from build123d import *

# Parameters (mm, degrees)
BOSS_EXTRUDE2_DEPTH = 18
SKETCH7_W           = 24
SKETCH7_H           = 13
CUT_EXTRUDE8_DEPTH  = 16.5


with BuildPart() as part:
    # Sketch2 → Boss-Extrude2 (new body)
    with BuildSketch(Plane(origin=(0, 0, 0), x_dir=(1, 0, 0), z_dir=(0, 1, 0))):
        with BuildLine():
            Line((14.142135624, 0), (48.904069139, 34.761933515))
            ThreePointArc((48.904069139, 34.761933515), (42.426406871, 42.426406871), (34.761933515, 48.904069139))
            Line((34.761933515, 48.904069139), (0, 14.142135624))
            Line((0, 14.142135624), (-34.761933515, 48.904069139))
            ThreePointArc((-34.761933515, 48.904069139), (-42.426406871, 42.426406871), (-48.904069139, 34.761933515))
            Line((-48.904069139, 34.761933515), (-14.142135624, 0))
            Line((-14.142135624, 0), (-48.904069139, -34.761933515))
            ThreePointArc((-48.904069139, -34.761933515), (-42.426406871, -42.426406871), (-34.761933515, -48.904069139))
            Line((-34.761933515, -48.904069139), (0, -14.142135624))
            Line((0, -14.142135624), (34.761933515, -48.904069139))
            ThreePointArc((34.761933515, -48.904069139), (42.426406871, -42.426406871), (48.904069139, -34.761933515))
            Line((48.904069139, -34.761933515), (14.142135624, 0))
        make_face()
    extrude(amount=BOSS_EXTRUDE2_DEPTH)

    # Sketch7 → Cut-Extrude8 (cut)
    with BuildSketch(Plane(origin=(0, 18, 0), x_dir=(1, 0, 0), z_dir=(0, 1, 0))):
        with Locations((5.6, 0)):
            Rectangle(SKETCH7_W, SKETCH7_H)
    extrude(amount=-CUT_EXTRUDE8_DEPTH, mode=Mode.SUBTRACT)


solid = part.part
Input: part model. Units: mm. Frame: model coordinates. A direction names the side the tool comes from. Give positions to 0.01 mm unless a question says otherwise; leave off trailing zeros. Order: outer loops, then holes, each group sorted by start corner. A loop starts at its lowest first (then second) coordinate and runs counter-clockwise, first axis right, second up.
Q1. Draft query along X for faces 5 (the cylindrical face through (-42.327, 8.874, -42.526)), 6 (the flat face through (-17.624, 8.874, 31.766)), 7 (the flat face through (-1, 0, -1)). Return one class per face: +X half, -X half, draft (parallel to the pull), parting line (faces both ways), or undercut.
Checked values:
face 5: -X half
face 6: undercut
face 7: draft
Q2. Ray query, probe 1 along Y at (x, z) = (2, 5); probe 2 along Z at (x, y) = (-15, 8.75); probe 3 along X at (y, z) = (15.5, -28.5). Return the intervals inside material, ascending.
Checked values:
probe 1: y = 0 to 1.5
probe 2: z = -29.14 to -0.86, 0.86 to 29.14
probe 3: x = -42.64 to -14.36, 14.36 to 42.64
Q3. Set-up query: faces 1 (the flat face through (-17.14, 8.87, -31.28)), 2 (the flat face through (-31.28, 8.87, 17.14)), 3 (the flat face through (5, 1.5, 0)), 4 (the flat face through (31.28, 8.87, -17.14)). Return all of +Z, -Z, +X, -X, +Y, -Y with unobstructed straight access to the full face (end or side cutting, diameter ignored); none if empty.
Checked values:
face 1: -Z, +Y, -Y
face 2: -X, +Y, -Y
face 3: +Y
face 4: +X, +Y, -Y
Q4. Contact query for flat-ended pins moving along their axis: pin 1 Ø1.5 at (y, z) = (7, 5) entering from -X; pin 2 Ø8 at (x, y) = (19, 13) entering from +Z; pin 3 Ø4 at (y, z) = (14, 16) entering from -X. Output: stop coordinate, or through.
Checked values:
pin 1: stops at x = -19.89
pin 2: stops at z = 37.14
pin 3: stops at x = -32.14
Q5. Section B-B on x = -39. Output: boundary loops of the cut face in (y, z).
Checked values:
outline: (0, -45.6) - (18, -45.6) - (18, -24.86) - (0, -24.86) - close; (0, 24.86) - (18, 24.86) - (18, 45.6) - (0, 45.6) - close
Q6. Section A-A on y = 2.75. Output: boundary loops of the cut face in (x, z).
Checked values:
outline: (-48.9, -34.76) arc R60 ccw to (-34.76, -48.9) - (0, -14.14) - (34.76, -48.9) arc R60 ccw to (48.9, -34.76) - (17.6, -3.46) - (17.6, -6.5) - (-6.4, -6.5) - (-6.4, 6.5) - (17.6, 6.5) - (17.6, 3.46) - (48.9, 34.76) arc R60 ccw to (34.76, 48.9) - (0, 14.14) - (-34.76, 48.9) arc R60 ccw to (-48.9, 34.76) - (-14.14, 0) - close
Q7. Section D-D on x = 7. Output: boundary loops of the cut face in (y, z).
Checked values:
outline: (0, -21.14) - (18, -21.14) - (18, -6.5) - (1.5, -6.5) - (1.5, 6.5) - (18, 6.5) - (18, 21.14) - (0, 21.14) - close
Q8. Section C-C on z = -19.5. Output: boundary loops of the cut face in (x, y).
Checked values:
outline: (-33.64, 0) - (-5.36, 0) - (-5.36, 18) - (-33.64, 18) - close; (5.36, 0) - (33.64, 0) - (33.64, 18) - (5.36, 18) - close
